from build123d import *

# Parameters (mm, degrees)
SKETCH2_R            = 15
BOSS_EXTRUDE1_DEPTH  = 6.35
M3_CLEARANCE_HOLE1_D = 3.4
CIRPATTERN1_COUNT    = 4
FILLET1_R            = 10


with BuildPart() as part:
    # Sketch2 → Boss-Extrude1 (new body)
    with BuildSketch(Plane(origin=(0, 0, 0), x_dir=(1, 0, 0), z_dir=(0, 1, 0))):
        with BuildLine():
            ThreePointArc((15, 0), (0, -15), (-15, 0))
            Line((-15, 0), (-15, -120))
            Line((-15, -120), (-65, -120))
            Line((-65, -120), (-65, -150))
            Line((-65, -150), (15, -150))
            Line((15, -150), (15, 0))
        make_face()
        Circle(SKETCH2_R)
    extrude(amount=BOSS_EXTRUDE1_DEPTH)

    # M3 Clearance Hole1 (through all)
    with Locations(Plane(origin=(0, 6.35, 0), x_dir=(1, 0, 0), z_dir=(0, 1, 0))):
        with Locations((0, 7)):
            m3_clearance_hole1 = Hole(M3_CLEARANCE_HOLE1_D / 2)

    # CirPattern1: M3 Clearance Hole1 ×4 about axis
    cirpattern1_axis = Axis((0, 0, 0), (0, 1, 0))
    for i in range(1, CIRPATTERN1_COUNT):
        add(m3_clearance_hole1.rotate(cirpattern1_axis, i * 360 / CIRPATTERN1_COUNT), mode=Mode.SUBTRACT)

    # Fillet1
    fillet1_edges = [part.edges().sort_by_distance(p)[0] for p in [
        (15, 3.175, 150),
        (-65, 3.175, 150),
        (-65, 3.175, 120),
        (-15, 3.175, 120),
    ]]
    fillet(fillet1_edges, radius=FILLET1_R)


solid = part.part
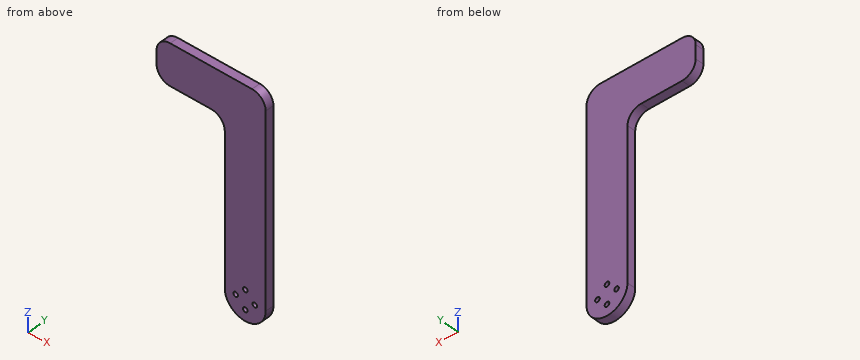
Geometry: final body of the model. Coordinates: model frame, mm. Round coordinates to 2 decimals unless told otherwise and drop trailing zeros. Order: outer loops, then holes, each group sorted by start corner. A loop starts at its lowest first (then second) coordinate and runs counter-clockwise, first axis right, second up.
Q1. Section D-D, the plane z = 90.5. Output: boundary loops of the cut face in (x, y).
Result sheet:
outline: (-15, 0) - (15, 0) - (15, 6.35) - (-15, 6.35) - close
Q2. Section A-A, the plane z = 7. Output: boundary loops of the cut face in (x, y), and give its area (3 significant figures).
Result sheet:
outline: (-15, 0) - (-1.7, 0) - (-1.7, 6.35) - (-15, 6.35) - close; (1.7, 0) - (15, 0) - (15, 6.35) - (1.7, 6.35) - close
area: 169 mm2
Q3. Section C-C, the plane x = 0. Output: boundary loops of the cut face in (y, z).
Result sheet:
outline: (0, -15) - (6.35, -15) - (6.35, -8.7) - (0, -8.7) - close; (0, -5.3) - (6.35, -5.3) - (6.35, 5.3) - (0, 5.3) - close; (0, 8.7) - (6.35, 8.7) - (6.35, 150) - (0, 150) - close
Q4. Material intervals for probe 1 along Z at (x, y) = (0, 2.5); probe 2 along X at (y, z) = (6.25, 10); probe 3 along Z at (x, y) = (-6.5, 1), sorted ascending.
Result sheet:
probe 1: z = -15 to -8.7, -5.3 to 5.3, 8.7 to 150
probe 2: x = -15 to 15
probe 3: z = -13.52 to -1.62, 1.62 to 150
Q5. Pin query (flat end, axial travel): pin 1 (4.5 mm diameter, centred on x = 0, z = -7, fed in from +Y); pin 2 (2 mm diameter, centred on x = -7, z = 0, fed in from +Y); pin 3 (1.5 mm diameter, centred on y = 1, z = 64, fed in from -X). Return the tip coordinate at first contact, or that it passes through.
Result sheet:
pin 1: stops at y = 6.35
pin 2: passes through
pin 3: stops at x = -15
Q6. Section B-B, the plane y = 3.5. Output: boundary loops of the cut face in (x, z), and give its area (3 significant figures).
Result sheet:
outline: (-65, 130) arc R10 ccw to (-55, 120) - (-25, 120) arc R10 cw to (-15, 110) - (-15, 0) arc R15 ccw to (15, 0) - (15, 140) arc R10 ccw to (5, 150) - (-55, 150) arc R10 ccw to (-65, 140) - close; hole circle Ø3.4 at (-7, 0); hole circle Ø3.4 at (0, -7); hole circle Ø3.4 at (0, 7); hole circle Ø3.4 at (7, 0)
area: 6,270 mm2
